Design review of the part built by this model. Coordinates are the model's own, in mm. A direction names the side the tool comes from. Give positions to 0.01 mm unless a question says otherwise; leave off trailing zeros. Write each loop counter-clockwise with the first axis right and the second up, starting at its lowest first coordinate (ties: lowest second). Pieces come first, ordered by that corner, then holes. Notation, with made-up numbers: (88, -8.5) - (119, -8.5) arc R24 cw to (119, 2.5) - close; hole circle Ø11 at (-27, 47.5). An arc over 180 degrees is marked (long way). Use a Markdown table: item, result. Add a question column.
Autodesk Fusion 360 part; units mm, degrees
sketch "Bottom front base" plane through (0, 0, 0) normal (0, 0, 1) x (1, 0, 0)
  line L0 (40, 60) -> (60, 60)
  line L1 (60, 60) -> (60, -60)
  line L2 (60, -60) -> (40, -60)
  line L3 (60, 0) -> (57.5, 0) construction
  line L4 (57.5, -60) -> (57.5, -6) construction
  line L5 (57.5, -6) -> (-12.5, -6) construction
  line L6 (-12.5, -6) -> (-12.5, -34) construction
  line L7 (-12.5, -34) -> (-30, -34)
  line L8 (-12.5, -34) -> (40, -34)
  line L9 (40, -34) -> (40, -60)
  line L10 (-30, -34) -> (-30, -60)
  arc A0 (-30, 60) -> (-30, -60) centre (15, 0) ccw
  line L11 (-30, 34) -> (-30, 60)
  line L12 (-12.5, 34) -> (40, 34)
  line L13 (-12.5, 34) -> (-30, 34)
  line L14 (40, 34) -> (40, 60)
  dimension "d1" = 120
  dimension "d3" = 2.5
  dimension "d4" = 54
  dimension "d5" = 70
  dimension "d6" = 28
  dimension "d9" = 70
extrude "Bottom front height" add sketch "Bottom front base" along normal blind 5
sketch "Connector hole" plane through (60, 0, 0) normal (1, 0, 0) x (0, 1, 0)
  line L0 (-60, 0) -> (60, 0)
  line L1 (60, 0) -> (60, 5)
  line L2 (60, 5) -> (-60, 5)
  line L3 (-60, 5) -> (-60, 0)
  line L4 (0, 0) -> (0, -0.1551)
  line L5 (0, 0) -> (0, 5) construction
  line L6 (30, 4) -> (-30, 4)
  line L7 (-30, 4) -> (-30, 1)
  line L8 (-30, 1) -> (30, 1)
  line L9 (30, 1) -> (30, 4)
  line L10 (30, 4) -> (-30, 1) construction
  line L11 (-30, 4) -> (30, 1) construction
  point P0 (0, 2.5)
  dimension "d12" = 3
  dimension "d13" = 60
extrude "Connector hole (1)" cut sketch "Connector hole" against normal blind 60 contours L6 L7 L8 L9
equation "d6 = 54 mm - 26 mm"
(1) Insertion check: pin 1 (1 mm diameter, centred on x = -42.5, z = 2, fed in from +Y); pin 2 (10 mm diameter, centred on x = -40.5, y = -5, fed in from -Z); pin 3 (1.5 mm diameter, centred on x = 29.5, z = 2, fed in from +Y); pin 4 (2.5 mm diameter, centred on y = 47, z = 2.5, fed in from -X). Each pin has a flat end and moves straight along its axis. Give the tip position at first contact, or say it passes through.
(2) Add section D-D (y = 52.5). State the section outline as (x, z) points, and give its area (3 significant figures).
(3) Add section C-C (y = 20). State the section outline as (x, z) points, and give its area (3 significant figures).
(4) Add section A-A (z = 2.95). State the section outline as (x, y) points, and give its area (3 significant figures).
(5) Add section B-B (x = 9). State the section outline as (y, z) points, and give its area (3 significant figures).
(6) Tool access review of faces 1 (the face through (-1, 1, 5)), 2 (the face through (0, 0, 3)), 3 (the face through (-30, -47, 2)), 4 (the face through (50, 60, 2)), 5 (the face through (40, 47, 2)): name each direction out of +Z, -Z, +X, -X, +Y, -Y from which nothing blocks a thin tool from reaching the whole face with its end or side.
(7) Mouldability with a two-part tool opening along X and no side actions: class faces 6 (the face through (60, 0.8, 0.8)), 7 (the face through (-59.994, -0.974, 2.465)), 8 (the face through (30, 0, 4)), 9 (the face through (-30, 47, 2)) as +X half, -X half, draft (parallel to the pull), parting line (faces both ways), or undercut.
(8) For line 1 along Z through (x, y) = (8.5, 7.5); line 2 along Y through (x, z) = (47, 3.35); line 3 along Y through (x, z) = (15, 1.45), list the stretches that pass through material, from the lowest coordinate up.
Answers follow:
| question | item | result |
|---|---|---|
| 1 | pin 1 | y = 48.74 |
| 1 | pin 2 | z = 0 |
| 1 | pin 3 | y = 34 |
| 1 | pin 4 | x = -44.43 |
| 2 | outline | (-38.56, 0) - (-30, 0) - (-30, 5) - (-38.56, 5) - close; (40, 0) - (60, 0) - (60, 5) - (40, 5) - close |
| 2 | area | 143 mm^2 |
| 3 | outline | (-57.28, 0) - (60, 0) - (60, 1) - (0, 1) - (0, 4) - (60, 4) - (60, 5) - (-57.28, 5) - close |
| 3 | area | 406 mm^2 |
| 4 | outline | (-30, -60) - (-30, -34) - (40, -34) - (40, -60) - (60, -60) - (60, -30) - (0, -30) - (0, 30) - (60, 30) - (60, 60) - (40, 60) - (40, 34) - (-30, 34) - (-30, 60) arc R75 ccw to start |
| 4 | area | 6,080 mm^2 |
| 5 | outline | (-34, 0) - (34, 0) - (34, 5) - (-34, 5) - close; hole (-30, 1) - (30, 1) - (30, 4) - (-30, 4) - close |
| 5 | area | 160 mm^2 |
| 6 | face 1 | +Z, +X, -X, +Y, -Y |
| 6 | face 2 | +X |
| 6 | face 3 | +Z, -Z, -Y |
| 6 | face 4 | +Z, -Z, +X, -X, +Y |
| 6 | face 5 | +Z, -Z, +Y |
| 7 | face 6 | +X half |
| 7 | face 7 | -X half |
| 7 | face 8 | draft |
| 7 | face 9 | undercut |
| 8 | line 1 | 0 to 1, 4 to 5 |
| 8 | line 2 | -60 to -30, 30 to 60 |
| 8 | line 3 | -34 to -30, 30 to 34 |
